from build123d import *

# Parameters (mm, degrees)
SKETCH2_R           = 762
BOSS_EXTRUDE1_DEPTH = 12.7
BOSS_EXTRUDE2_DEPTH = 25.4
BOSS_EXTRUDE3_DEPTH = 25.4
FILLET1_R           = 50.8
FILLET2_R           = 50.8
FILLET3_R           = 2.54


with BuildPart() as part:
    # Sketch2 → Boss-Extrude1 (new body)
    with BuildSketch(Plane(origin=(0, 0, 0), x_dir=(1, 0, 0), z_dir=(0, 1, 0))):
        with Locations(Location((0, 0, 0), (0, 0, 270))):
            Circle(SKETCH2_R)
    extrude(amount=BOSS_EXTRUDE1_DEPTH)

    # Sketch3 → Boss-Extrude2 (add, symmetric)
    with BuildSketch(Plane(origin=(0, 0, 0), x_dir=(0, 0, -1), z_dir=(1, 0, 0))):
        with BuildLine():
            Line((-376.512914222, 0), (-519.686562072, 0))
            Line((-519.686562072, 0), (-222.871959454, -142.716140502))
            ThreePointArc((-222.871959454, -142.716140502), (-182.701733049, -190.186232292), (-191.275920014, -251.777952693))
            Line((-191.275920014, -251.777952693), (-489.061959381, -728.203177114))
            Line((-489.061959381, -728.203177114), (-476.851322016, -728.203177114))
            Line((-476.851322016, -728.203177114), (0, -205.292352404))
            Line((0, -205.292352404), (476.851322016, -728.203177114))
            Line((476.851322016, -728.203177114), (489.061959381, -728.203177114))
            Line((489.061959381, -728.203177114), (191.275920014, -251.777952693))
            ThreePointArc((191.275920014, -251.777952693), (182.701733049, -190.186232292), (222.871959454, -142.716140502))
            Line((222.871959454, -142.716140502), (519.686562072, 0))
            Line((519.686562072, 0), (376.512914222, 0))
            Line((376.512914222, 0), (0, -97.717234055))
            Line((0, -97.717234055), (-376.512914222, 0))
        make_face()
    extrude(amount=BOSS_EXTRUDE2_DEPTH, both=True)

    # Sketch5 → Boss-Extrude3 (add, symmetric)
    with BuildSketch(Plane.XY):
        with BuildLine():
            Line((-547.036781798, 0.405352419), (-249.591046968, -142.614252779))
            ThreePointArc((-249.591046968, -142.614252779), (-209.420820563, -190.08434457), (-217.995007528, -251.676064971))
            Line((-217.995007528, -251.676064971), (-512.749991198, -723.251930457))
            Line((-512.749991198, -723.251930457), (-499.148196201, -723.251930457))
            Line((-499.148196201, -723.251930457), (-3.147209779, -179.341757847))
            Line((-3.147209779, -179.341757847), (-3.147209779, -103.733008189))
            Line((-3.147209779, -103.733008189), (-404.401277334, 0.405352419))
            Line((-404.401277334, 0.405352419), (-547.036781798, 0.405352419))
        make_face()
        with BuildLine():
            ThreePointArc((249.591046968, -142.614252779), (209.420820563, -190.08434457), (217.995007528, -251.676064971))
            Line((217.995007528, -251.676064971), (512.749991198, -723.251930457))
            Line((512.749991198, -723.251930457), (499.148196201, -723.251930457))
            Line((499.148196201, -723.251930457), (3.147209779, -179.341757847))
            Line((3.147209779, -179.341757847), (3.147209779, -103.733008189))
            Line((3.147209779, -103.733008189), (404.401277334, 0.405352419))
            Line((404.401277334, 0.405352419), (547.036781798, 0.405352419))
            Line((547.036781798, 0.405352419), (249.591046968, -142.614252779))
        make_face()
    extrude(amount=BOSS_EXTRUDE3_DEPTH, both=True)

    # Fillet1
    fillet1_edges = [part.edges().sort_by_distance(p)[0] for p in [
        (25.4, -150.850828677, 25.4),
    ]]
    fillet(fillet1_edges, radius=FILLET1_R)

    # Fillet2
    fillet2_edges = [part.edges().sort_by_distance(p)[0] for p in [
        (-25.4, -150.850828677, -25.4),
        (-25.4, -150.850828677, 25.4),
        (25.4, -150.850828677, -25.4),
    ]]
    fillet(fillet2_edges, radius=FILLET2_R)

    # Fillet3
    fillet3_edges = [part.edges().sort_by_distance(p)[0] for p in [
        (-25.4, -489.990564904, 340.168939697),
        (25.4, -489.990564904, -340.168939697),
        (25.4, -190.186232292, -182.701733049),
        (25.4, -71.358070251, -371.279260763),
        (25.4, -71.358070251, 371.279260763),
        (25.4, -190.186232292, 182.701733049),
        (25.4, -489.990564904, 340.168939697),
        (-25.4, -71.358070251, -371.279260763),
        (-25.4, -190.186232292, -182.701733049),
        (-25.4, -489.990564904, -340.168939697),
        (-397.892397529, -71.30712639, -25.4),
        (-397.892397529, -71.30712639, 25.4),
        (-209.420820563, -190.08434457, 25.4),
        (-365.372499363, -487.463997714, 25.4),
        (-209.420820563, -190.08434457, -25.4),
        (-365.372499363, -487.463997714, -25.4),
        (397.892397529, -71.30712639, 25.4),
        (397.892397529, -71.30712639, -25.4),
        (209.420820563, -190.08434457, -25.4),
        (365.372499363, -487.463997714, -25.4),
        (209.420820563, -190.08434457, 25.4),
        (365.372499363, -487.463997714, 25.4),
        (-25.4, -71.358070251, 371.279260763),
        (-25.4, -190.186232292, 182.701733049),
    ]]
    fillet(fillet3_edges, radius=FILLET3_R)


solid = part.part
Design review of the part built by this model. Coordinates are the model's own, in mm. A direction names the side the tool comes from. Coordinates: 2 decimals unless noted, no trailing zeros. Order: outer loops, then holes, each group sorted by start corner. A loop starts at its lowest first (then second) coordinate and runs counter-clockwise, first axis right, second up. Notation, with made-up numbers: (16, 31.5) -> (59, 31.5) arc R24 cw to (59, 70.5) -> close; hole circle Ø6 at (55, -26.75). An arc over 180 degrees is marked (long way). Use one line per item in the form item = value. Start each with the question number.
(1) Add section C-C on z = -580. State the section outline as (x, y) points, plus the area to 3 significant figures.
(2) Add section D-D on x = 620.5. State the section outline as (y, z) points.
(3) The part is to be moulded in two halves that separate along Z. For faces 1 (the cylindrical face through (47.52, -151.48, -34.27)), 2 (the cylindrical face through (-46.607, -153.926, 34.91)), 3 (the flat face through (0.356, -470.408, 241.764)), say which applies: +Z half, -Z half, draft (parallel to the pull), parting line (faces both ways), or undercut.
(4) Insertion check: pin 1 (11 mm diameter, centred on x = -509.5, z = 8, fed in from -Y); pin 2 (5 mm diameter, centred on x = -457, z = -62, fed in from -Y); pin 3 (3 mm diameter, centred on y = -404, z = -238, fed in from +X); pin 4 (8 mm diameter, centred on x = 234.5, y = -264, fed in from -Z). Each pin has a flat end and moves straight along its axis. Give the tip position at first contact, or say it passes through.
(5) For probe 1 along Y at (x, z) = (-608, -321); probe 2 along X at (y, z) = (-218, -97.5); probe 3 along Z at (x, y) = (-58, -214), list the stretches that pass through material, from the lowest coordinate up.
(6) For faces 4 (the flat face through (223, -280, 25.4)), 5 (the flat face through (0.32, -70.359, 373.357)), 6 (the cylindrical face through (24.676, -487.06, -337.437)), list the 3-axis set-ups (+Z, -Z, +X, -X, +Y, -Y) from which the entire face can be reached by the end or side of a thin tool; tool diameter is ignored.
(7) Add section A-A on x = 0. State the section outline as (y, z) points, plus the area to 3 significant figures.
(8) Add section B-B on y = -374. Give the number of separate pieces and of enclosed holes in the cut face, plus the area to 3 significant figures.
Answer block:
q1.outline = (-494.21, 0) -> (494.21, 0) -> (494.21, 12.7) -> (-494.21, 12.7) -> close
q1.area = 12,600 mm²
q2.outline = (0, -442.29) -> (12.7, -442.29) -> (12.7, 442.29) -> (0, 442.29) -> close
q3.face_1 = -Z half
q3.face_2 = +Z half
q3.face_3 = undercut
q4.pin_1 = -723.25
q4.pin_2 = 0
q4.pin_3 = 25.4
q4.pin_4 = through
q5.probe_1 = 0 to 12.7
q5.probe_2 = -25.4 to 25.4
q5.probe_3 = -28.77 to 28.77
q6.face_4 = +Z, +X, -Y
q6.face_5 = +Z, +X, -X
q6.face_6 = -Z, +X
q7.outline = (-728.2, -489.06) -> (-251.78, -191.28) arc R76.2 cw to (-142.72, -222.87) -> (0, -519.69) -> (0, -762) -> (12.7, -762) -> (12.7, 762) -> (0, 762) -> (0, 519.69) -> (-142.72, 222.87) arc R76.2 cw to (-251.78, 191.28) -> (-728.2, 489.06) -> (-728.2, 476.85) -> (-205.29, 0) -> (-728.2, -476.85) -> close; hole (-97.72, 0) -> (0, -376.51) -> (0, 376.51) -> close
q7.area = 204,000 mm²
q8.separate_pieces = 4
q8.enclosed_holes = 0
q8.area = 23,100 mm²
